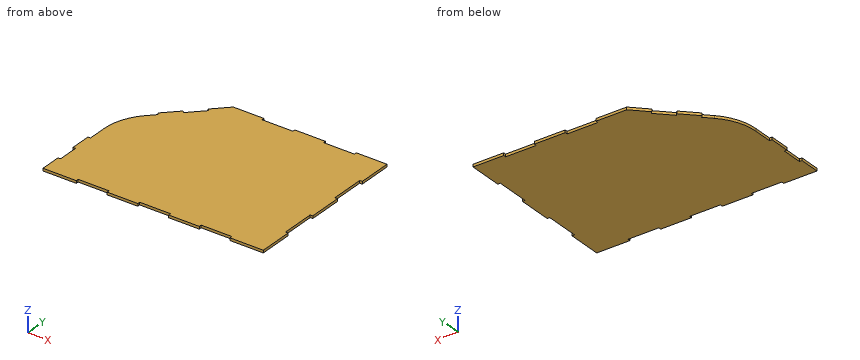
from build123d import *

# Parameters (mm, degrees)
BOSS_EXTRU_1_DEPTH      = 5
ENL_V_MAT_EXTRU_1_REACH = 7


with BuildPart() as part:
    # Esquisse1 → Boss.-Extru.1 (new body)
    with BuildSketch(Plane.XY):
        Polygon((0, 330), (-60, 330), (-60, 325), (-120, 325), (-120, 330), (-180, 330), (-180, 325), (-240, 325), (-240, 330), (-300, 330), (-328.284271247, 301.715728753), (-324.748737342, 298.180194847), (-353.033008589, 269.895923599), (-356.568542495, 273.431457505), (-399.901875828, 230.098124172), (-396.366341922, 226.562590266), (-411.415404008, 211.51352818), (-414.950937914, 215.049062086), (-430, 200), (-430, 160), (-425, 160), (-425, 120), (-430, 120), (-430, 80), (-425, 80), (-425, 40), (-430, 40), (-430, 0), (-365, 0), (-365, 5), (-305, 5), (-305, 0), (-245, 0), (-245, 5), (-185, 5), (-185, 0), (-125, 0), (-125, 5), (-65, 5), (-65, 0), (0, 0), (0, 66), (-5, 66), (-5, 132), (0, 132), (0, 198), (-5, 198), (-5, 264), (0, 264), align=None)
    extrude(amount=BOSS_EXTRU_1_DEPTH)

    # Esquisse2 → Enlèv. mat.-Extru.1 (cut, up to next)
    with BuildSketch(Plane.XY.offset(5), mode=Mode.PRIVATE) as enl_v_mat_extru_1_sk1:
        with BuildLine():
            Line((-395.710678119, 227.218254069), (-381.568542495, 241.360389693))
            Line((-381.568542495, 241.360389693), (-385.104076401, 244.895923599))
            Line((-385.104076401, 244.895923599), (-430, 200))
            Line((-430, 200), (-430, 156.507575951))
            Line((-430, 156.507575951), (-425, 156.507575951))
            ThreePointArc((-425, 156.507575951), (-417.387953251, 194.775919187), (-395.710678119, 227.218254069))
        make_face()
    enl_v_mat_extru_1_tool1 = extrude(enl_v_mat_extru_1_sk1.sketch, amount=-ENL_V_MAT_EXTRU_1_REACH, mode=Mode.PRIVATE) & part.part
    add(enl_v_mat_extru_1_tool1.solids().sort_by_distance((-415.711514, 201.173028, 5))[0], mode=Mode.SUBTRACT)


solid = part.part
Work out the finished part from the listing and answer in its coordinate system (mm). Give positions to 0.01 mm unless a question says otherwise; leave off trailing zeros. Loops run counter-clockwise (first coordinate to the right, second up) from the corner with the lowest first, then second, coordinate; pieces in that order, holes last. Notation, with made-up numbers: (89, 60.25) -> (133, 60.25) arc R15 cw to (133, 71.25) -> close; hole circle Ø10 at (33, -7). An arc over 180 degrees is marked (long way). Use a Markdown table: item, result. Add a question column.
1) The part is cut by section A-A, the plane y = 75.5. Determine the outline of the cut face in (x, z).
2) Each of these flat-tipped pins is pushed along its axis until it touches: P1, Ø1.5, axis at y = 328.5, z = 3.5, coming from the -X side; P2, Ø2, axis at x = -350, z = 3, coming from the -Y side; P3, Ø1.5, axis at y = 90, z = 2, coming from the +X side. Where does it stop, or does it pass through?
3) The part is cut by section B-B, the plane x = -199. Determine the outline of the cut face in (y, z), plus the area to 3 significant figures.
4) Consider line 1 along X through (y, z) = (107.5, 4); line 2 along X through (y, z) = (55, 4.3); line 3 along Y through (x, z) = (-78.5, 4.4). Determine where each line is inside the solid, lowest interval first.
Reported:
| question | item | result |
|---|---|---|
| 1 | outline | (-425, 0) -> (-5, 0) -> (-5, 5) -> (-425, 5) -> close |
| 2 | P1 | stops at x = -302.25 |
| 2 | P2 | stops at y = 5 |
| 2 | P3 | stops at x = -5 |
| 3 | outline | (5, 0) -> (325, 0) -> (325, 5) -> (5, 5) -> close |
| 3 | area | 1,600 mm^2 |
| 4 | line 1 | x = -430 to -5 |
| 4 | line 2 | x = -425 to 0 |
| 4 | line 3 | y = 5 to 325 |
